Read the model definition and answer for the solid it produces. Units are mm, in the model's axes. A direction names the side the tool comes from. Round coordinates to 2 decimals unless told otherwise and drop trailing zeros. Loops run counter-clockwise (first coordinate to the right, second up) from the corner with the lowest first, then second, coordinate; pieces in that order, holes last. Notation, with made-up numbers: (-26.75, -25.75) -> (-19.75, -25.75) arc R13 cw to (-19.75, -20.75) -> close; hole circle Ø4 at (59.25, -28). An arc over 180 degrees is marked (long way). Put each result on its own line as item: value.
from build123d import *

# Parameters (mm, degrees)
BOSS_EXTRUDE1_DEPTH = 10
SKETCH2_R           = 2.25
BOSS_EXTRUDE2_DEPTH = 4


with BuildPart() as part:
    # Sketch1 → Boss-Extrude1 (new body)
    with BuildSketch(Plane(origin=(0, 0, 0), x_dir=(1, 0, 0), z_dir=(0, 1, 0))):
        Polygon((0, -40), (0, 0), (-3, 0), (-3, -43), (63, -43), (63, 0), (60, 0), (60, -40), align=None)
    extrude(amount=BOSS_EXTRUDE1_DEPTH)

    # Sketch2 → Boss-Extrude2 (add)
    with BuildSketch(Plane(origin=(0, 0, 0), x_dir=(1, 0, 0), z_dir=(0, 1, 0))):
        with BuildLine():
            Line((0, -15), (0, -25))
            Line((0, -25), (21.339745962, -25))
            ThreePointArc((21.339745962, -25), (22.928932188, -27.071067812), (25, -28.660254038))
            Line((25, -28.660254038), (25, -40))
            Line((25, -40), (35, -40))
            Line((35, -40), (35, -28.660254038))
            ThreePointArc((35, -28.660254038), (37.071067812, -27.071067812), (38.660254038, -25))
            Line((38.660254038, -25), (60, -25))
            Line((60, -25), (60, -15))
            Line((60, -15), (38.660254038, -15))
            ThreePointArc((38.660254038, -15), (30, -10), (21.339745962, -15))
            Line((21.339745962, -15), (0, -15))
        make_face()
        with Locations(Location((30, -20, 0), (0, 0, 270))):
            Circle(SKETCH2_R, mode=Mode.SUBTRACT)
    extrude(amount=BOSS_EXTRUDE2_DEPTH)


solid = part.part
Item 1: Which of the six approach directions +Z, -Z, +X, -X, +Y, -Y give full straight-line access (tool end or side, diameter ignored) to faces 4 (the flat face through (49, 2, 15)), 5 (the cylindrical face through (37.045, 1.972, 27.097)), 6 (the flat face through (30, 10, 41)), 7 (the flat face through (0, 5, 20)), 8 (the flat face through (30, 5, 43))?
Derived:
face 4: -Z, +Y, -Y
face 5: +Y, -Y
face 6: +Z, -Z, +X, -X, +Y
face 7: +Y
face 8: +Z, +X, -X, +Y, -Y
Item 2: For a pull along X with two mould halves and no side action, classify faces 1 (the flat face through (-3, 5, 21)), 2 (the flat face through (-1, 5, 0)), 3 (the flat face through (49, 2, 25)) as pulls with the +X half, pulls with the -X half, needs draft (parallel to the pull), parting line crosses it, or undercut.
Derived:
face 1: pulls with the -X half
face 2: needs draft
face 3: undercut
Item 3: The part is cut by section D-D (y = 5.5). Determine the outline of the cut face in (x, z).
Derived:
outline: (-3, 0) -> (0, 0) -> (0, 40) -> (60, 40) -> (60, 0) -> (63, 0) -> (63, 43) -> (-3, 43) -> close
Item 4: The part is cut by section C-C (z = 38.5). Determine the outline of the cut face in (x, y), then the cut area to 3 significant figures.
Derived:
outline: (-3, 0) -> (0, 0) -> (0, 10) -> (-3, 10) -> close; (25, 0) -> (35, 0) -> (35, 4) -> (25, 4) -> close; (60, 0) -> (63, 0) -> (63, 10) -> (60, 10) -> close
area: 100 mm^2
Item 5: The part is cut by section A-A (z = 20). Determine the outline of the cut face in (x, y).
Derived:
outline: (-3, 0) -> (27.75, 0) -> (27.75, 4) -> (0, 4) -> (0, 10) -> (-3, 10) -> close; (32.25, 0) -> (63, 0) -> (63, 10) -> (60, 10) -> (60, 4) -> (32.25, 4) -> close
Item 6: Find the intervals of material crossed by line 1 along X through (y, z) = (2.5, 20); line 2 along X through (y, z) = (7, 37); line 3 along Z through (x, y) = (1, 1.5), in increasing order.
Derived:
line 1: x = -3 to 27.75, 32.25 to 63
line 2: x = -3 to 0, 60 to 63
line 3: z = 15 to 25, 40 to 43
Item 7: Flat-ended cylindrical pins translate along their axes: pin 1 Ø3 at (x, y) = (52.5, 2) entering from -Z; pin 2 Ø10 at (x, z) = (14.5, 20) entering from +Y; pin 3 Ø4 at (x, z) = (30, 20) entering from +Y. Find the tip coordinate at first contact, or state that the pin passes through.
Derived:
pin 1: stops at z = 15
pin 2: stops at y = 4
pin 3: passes through
Item 8: The part is cut by section B-B (x = 30). Determine the outline of the cut face in (y, z).
Derived:
outline: (0, 10) -> (4, 10) -> (4, 17.75) -> (0, 17.75) -> close; (0, 22.25) -> (4, 22.25) -> (4, 40) -> (10, 40) -> (10, 43) -> (0, 43) -> close
